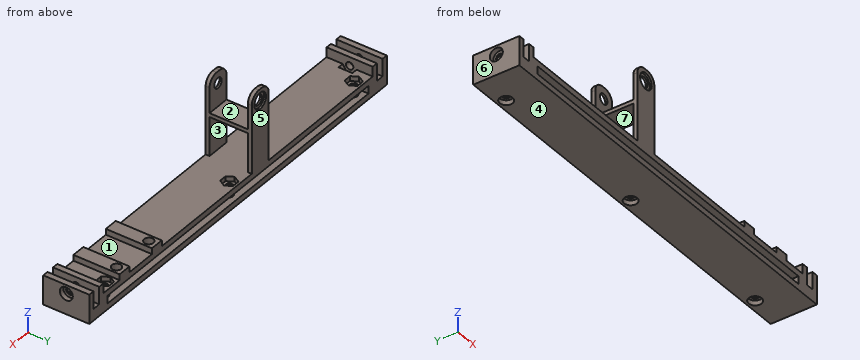
```python
from build123d import *

# Parameters (mm, degrees)
SKETCH2_W            = 23.75
SKETCH2_H            = 12
BOSS_EXTRUDE1_DEPTH  = 10
SKETCH3_W            = 12
SKETCH3_H            = 2.025
BOSS_EXTRUDE2_DEPTH  = 40
FILLET1_R            = 5
FILLET1_OF_MIRROR1_R = 5
SKETCH5_R            = 2.65
CUT_EXTRUDE1_DEPTH   = 57.639760769
SKETCH6_R            = 4.15
CUT_EXTRUDE2_DEPTH   = 1
SKETCH7_W            = 84
SKETCH7_H            = 23.75
SKETCH7_W_2          = 115.5
BOSS_EXTRUDE3_DEPTH  = 10
SKETCH8_W            = 10
SKETCH8_H            = 23.75
BOSS_EXTRUDE4_DEPTH  = 5
BOSS_EXTRUDE7_REACH  = 130.079
SKETCH18_W           = 12
SKETCH18_H           = 2
SKETCH11_W           = 185.5
SKETCH11_H           = 4
CUT_EXTRUDE3_DEPTH   = 9
SKETCH12_R           = 1.9
CUT_EXTRUDE4_DEPTH   = 155.807138078
SKETCH15_R           = 3.35
CUT_EXTRUDE5_DEPTH   = 2.5
SKETCH16_R           = 1.9
CUT_EXTRUDE6_DEPTH   = 2.5
LPATTERN1_COUNT      = 3
LPATTERN1_PITCH      = 88.5
SKETCH14_W           = 7
SKETCH14_H           = 23.75
BOSS_EXTRUDE6_DEPTH  = 3
CUT_EXTRUDE7_REACH   = 130.079
SKETCH21_W           = 4
SKETCH21_H           = 9
LPATTERN2_COUNT      = 2
LPATTERN2_PITCH      = 201.5
SKETCH22_R           = 2.4
CUT_EXTRUDE8_DEPTH   = 3.8
SKETCH26_R           = 1.75
CUT_EXTRUDE12_DEPTH  = 0.6
LPATTERN3_COUNT      = 2
LPATTERN3_PITCH      = 23
SKETCH23_R           = 1.9
CUT_EXTRUDE9_DEPTH   = 10
SKETCH24_R           = 3.35
CUT_EXTRUDE10_DEPTH  = 2.5
CUT_EXTRUDE11_DEPTH  = 3


with BuildPart() as part:
    # Sketch2 → Boss-Extrude1 (new body)
    with BuildSketch(Plane(origin=(0, 0, 0), x_dir=(0, 1, 0), z_dir=(0, 0, 1))):
        with Locations((-83.125, 6)):
            Rectangle(SKETCH2_W, SKETCH2_H)
    extrude(amount=BOSS_EXTRUDE1_DEPTH)

    # Sketch3 → Boss-Extrude2 (add)
    with BuildSketch(Plane.XY.offset(10)):
        with Locations((-6, -72.2625)):
            Rectangle(SKETCH3_W, SKETCH3_H)
    boss_extrude2 = extrude(amount=BOSS_EXTRUDE2_DEPTH)

    # Fillet1
    fillet1_edges = [part.edges().sort_by_distance(p)[0] for p in [
        (-12, -72.2625, 50),
        (0, -72.2625, 50),
    ]]
    fillet(fillet1_edges, radius=FILLET1_R)

    # Mirror1: Boss-Extrude2 across plane
    add(boss_extrude2.mirror(Plane.ZX.offset(-83.125)))

    # Fillet1 of Mirror1
    fillet1_of_mirror1_edges = [part.edges().sort_by_distance(p)[0] for p in [
        (-12, -93.9875, 50),
        (0, -93.9875, 50),
    ]]
    fillet(fillet1_of_mirror1_edges, radius=FILLET1_OF_MIRROR1_R)

    # Sketch5 → Cut-Extrude1 (cut, through all)
    with BuildSketch(Plane.XZ.offset(95)):
        with Locations(Location((-6, 44, 0), (0, 0, 270))):
            Circle(SKETCH5_R)
    extrude(amount=-CUT_EXTRUDE1_DEPTH, mode=Mode.SUBTRACT)

    # Sketch6 → Cut-Extrude2 (cut)
    with BuildSketch(Plane.XZ.offset(95)):
        with Locations(Location((-6, 44, 0), (0, 0, 270))):
            Circle(SKETCH6_R)
    cut_extrude2 = extrude(amount=-CUT_EXTRUDE2_DEPTH, mode=Mode.SUBTRACT)

    # Mirror2: Cut-Extrude2 across plane
    add(cut_extrude2.mirror(Plane.ZX.offset(-83.125)), mode=Mode.SUBTRACT)

    # Sketch7 → Boss-Extrude3 (add)
    with BuildSketch(Plane(origin=(0, 0, 0), x_dir=(1, 0, 0), z_dir=(0, 0, -1))):
        with Locations((-54, 83.125)):
            Rectangle(SKETCH7_W, SKETCH7_H)
        with Locations((57.75, 83.125)):
            Rectangle(SKETCH7_W_2, SKETCH7_H)
    extrude(amount=-BOSS_EXTRUDE3_DEPTH)

    # Sketch8 → Boss-Extrude4 (add)
    with BuildSketch(Plane.XY.offset(10)):
        with Locations((110.5, -83.125)):
            Rectangle(SKETCH8_W, SKETCH8_H)
        with Locations((-91, -83.125)):
            Rectangle(SKETCH8_W, SKETCH8_H)
    extrude(amount=BOSS_EXTRUDE4_DEPTH)

    # Sketch18 → Boss-Extrude7 (add, up to next)
    with BuildSketch(Plane(origin=(0, -71.25, 0), x_dir=(-1, 0, 0), z_dir=(0, 1, 0)), mode=Mode.PRIVATE) as boss_extrude7_sk1:
        with Locations((6, 31)):
            Rectangle(SKETCH18_W, SKETCH18_H)
    boss_extrude7_tool1 = extrude(boss_extrude7_sk1.sketch, amount=-BOSS_EXTRUDE7_REACH, mode=Mode.PRIVATE) - part.part
    add(boss_extrude7_tool1.solids().sort_by_distance((-6, -71.25, 31))[0])

    # Sketch11 → Cut-Extrude3 (cut)
    with BuildSketch(Plane(origin=(0, -71.25, 0), x_dir=(-1, 0, 0), z_dir=(0, 1, 0))):
        with Locations((-9.75, 5)):
            Rectangle(SKETCH11_W, SKETCH11_H)
    cut_extrude3 = extrude(amount=-CUT_EXTRUDE3_DEPTH, mode=Mode.SUBTRACT)

    # Mirror3: Cut-Extrude3 across plane
    add(cut_extrude3.mirror(Plane.ZX.offset(-83.125)), mode=Mode.SUBTRACT)

    # Sketch12 → Cut-Extrude4 (cut, symmetric)
    with BuildSketch(Plane.XY.offset(10)):
        with Locations((-78.75, -75.75)):
            Circle(SKETCH12_R)
    cut_extrude4 = extrude(amount=CUT_EXTRUDE4_DEPTH, both=True, mode=Mode.SUBTRACT)

    # Sketch15 → Cut-Extrude5 (cut)
    with BuildSketch(Plane.XY):
        with Locations((-78.75, -75.75)):
            Circle(SKETCH15_R)
    cut_extrude5 = extrude(amount=CUT_EXTRUDE5_DEPTH, mode=Mode.SUBTRACT)

    # Sketch16 → Cut-Extrude6 (cut)
    # profile 1 of 2: a face of its own
    with BuildSketch(Plane.XY.offset(10)):
        Polygon((-76.826794919, -72.418911087), (-80.673205081, -72.418911087), (-82.596410162, -75.75), (-80.673205081, -79.081088913), (-76.826794919, -79.081088913), (-74.903589838, -75.75), align=None)
        Polygon((-80.5, -72.718911087), (-82.25, -75.75), (-80.5, -78.781088913), (-77, -78.781088913), (-75.25, -75.75), (-77, -72.718911087), align=None, mode=Mode.SUBTRACT)
    # profile 2 of 2: a face of its own
    with BuildSketch(Plane.XY.offset(10)):
        Polygon((-77, -72.718911087), (-80.5, -72.718911087), (-82.25, -75.75), (-80.5, -78.781088913), (-77, -78.781088913), (-75.25, -75.75), align=None)
        with Locations((-78.75, -75.75)):
            Circle(SKETCH16_R, mode=Mode.SUBTRACT)
    cut_extrude6 = extrude(amount=-CUT_EXTRUDE6_DEPTH, mode=Mode.SUBTRACT)

    # LPattern1: Cut-Extrude4, Cut-Extrude5, Cut-Extrude6 ×3
    with Locations(*[(i * LPATTERN1_PITCH, 0, 0) for i in range(1, LPATTERN1_COUNT)]):
        add(cut_extrude4, mode=Mode.SUBTRACT)
        add(cut_extrude5, mode=Mode.SUBTRACT)
        add(cut_extrude6, mode=Mode.SUBTRACT)

    # Sketch14 → Boss-Extrude6 (add)
    with BuildSketch(Plane.XY.offset(10)):
        with Locations((67.5, -83.125)):
            Rectangle(SKETCH14_W, SKETCH14_H)
        with Locations((90.5, -83.125)):
            Rectangle(SKETCH14_W, SKETCH14_H)
    extrude(amount=BOSS_EXTRUDE6_DEPTH)

    # Sketch21 → Cut-Extrude7 (cut, up to next)
    with BuildSketch(Plane(origin=(0, -71.25, 0), x_dir=(-1, 0, 0), z_dir=(0, 1, 0)), mode=Mode.PRIVATE) as cut_extrude7_sk1:
        with Locations((-110.5, 10.5)):
            Rectangle(SKETCH21_W, SKETCH21_H)
    cut_extrude7_tool1 = extrude(cut_extrude7_sk1.sketch, amount=-CUT_EXTRUDE7_REACH, mode=Mode.PRIVATE) & part.part
    cut_extrude7 = cut_extrude7_tool1.solids().sort_by_distance((110.5, -71.25, 10.5))[0]
    add(cut_extrude7, mode=Mode.SUBTRACT)

    # LPattern2: Cut-Extrude7 ×2
    with Locations(*[(-i * LPATTERN2_PITCH, 0, 0) for i in range(1, LPATTERN2_COUNT)]):
        add(cut_extrude7, mode=Mode.SUBTRACT)

    # Sketch22 → Cut-Extrude8 (cut)
    with BuildSketch(Plane.XY.offset(13)):
        with Locations((90.5, -75.37)):
            Circle(SKETCH22_R)
    cut_extrude8 = extrude(amount=-CUT_EXTRUDE8_DEPTH, mode=Mode.SUBTRACT)

    # Sketch26 → Cut-Extrude12 (cut)
    with BuildSketch(Plane.XY.offset(9.2)):
        with Locations((90.5, -75.37)):
            Circle(SKETCH26_R)
    cut_extrude12 = extrude(amount=-CUT_EXTRUDE12_DEPTH, mode=Mode.SUBTRACT)

    # LPattern3: Cut-Extrude8, Cut-Extrude12 ×2
    with Locations(*[(-i * LPATTERN3_PITCH, 0, 0) for i in range(1, LPATTERN3_COUNT)]):
        add(cut_extrude8, mode=Mode.SUBTRACT)
        add(cut_extrude12, mode=Mode.SUBTRACT)

    # Sketch23 → Cut-Extrude9 (cut)
    with BuildSketch(Plane.YZ.offset(115.5)):
        with Locations(Location((-83.125, 10.5, 0), (0, 0, 270))):
            Circle(SKETCH23_R)
    cut_extrude9 = extrude(amount=-CUT_EXTRUDE9_DEPTH, mode=Mode.SUBTRACT)

    # Sketch24 → Cut-Extrude10 (cut)
    with BuildSketch(Plane.YZ.offset(115.5)):
        with Locations(Location((-83.125, 10.5, 0), (0, 0, 270))):
            Circle(SKETCH24_R)
    cut_extrude10 = extrude(amount=-CUT_EXTRUDE10_DEPTH, mode=Mode.SUBTRACT)

    # Sketch25 → Cut-Extrude11 (cut)
    with BuildSketch(Plane(origin=(105.5, 0, 0), x_dir=(0, -1, 0), z_dir=(-1, 0, 0))):
        Polygon((81.201794919, 13.831088913), (79.278589838, 10.5), (81.201794919, 7.168911087), (85.048205081, 7.168911087), (86.971410162, 10.5), (85.048205081, 13.831088913), align=None)
    cut_extrude11 = extrude(amount=CUT_EXTRUDE11_DEPTH, mode=Mode.SUBTRACT)

    # Mirror4: Cut-Extrude9, Cut-Extrude10, Cut-Extrude11 across plane
    add(cut_extrude9.mirror(Plane(origin=(9.75, 0, 0), x_dir=(0, 0, 1), z_dir=(1, 0, 0))), mode=Mode.SUBTRACT)
    add(cut_extrude10.mirror(Plane(origin=(9.75, 0, 0), x_dir=(0, 0, 1), z_dir=(1, 0, 0))), mode=Mode.SUBTRACT)
    add(cut_extrude11.mirror(Plane(origin=(9.75, 0, 0), x_dir=(0, 0, 1), z_dir=(1, 0, 0))), mode=Mode.SUBTRACT)


solid = part.part
```
Read the model definition and answer for the solid it produces. Units are mm, in the model's axes. Face numbers are marked on the shaded views. A direction names the side the tool comes from. Coordinates: 2 decimals unless noted, no trailing zeros. Write each loop counter-clockwise with the first axis right and the second up, starting at its lowest first coordinate (ties: lowest second). Pieces come first, ordered by that corner, then holes. Notation, with made-up numbers: (41.5, 9) -> (57.5, 9) arc R5 cw to (57.5, 13) -> close; hole circle Ø11 at (-26.5, 23). An arc over 180 degrees is marked (long way). Return JSON: item names as keys, results as strings.
1. A cutting plane is placed at C-C (x = -59). Determine the outline of the cut face in (y, z).
Found:
{"outline": "(-95, 0) -> (-71.25, 0) -> (-71.25, 3) -> (-80.25, 3) -> (-80.25, 7) -> (-71.25, 7) -> (-71.25, 10) -> (-95, 10) -> (-95, 7) -> (-86, 7) -> (-86, 3) -> (-95, 3) -> close"}
2. A cutting plane is placed at A-A (y = -90). Give the number of separate pieces and of enclosed holes in the cut face, and give its area (3 significant figures).
Found:
{"separate pieces": "2", "enclosed holes": "1", "area": "1,470 mm2"}
3. A cutting plane is placed at D-D (x = 90.5). Determine the outline of the cut face in (y, z), and give its area (3 significant figures).
Found:
{"outline": "(-95, 0) -> (-71.25, 0) -> (-71.25, 3) -> (-80.25, 3) -> (-80.25, 7) -> (-71.25, 7) -> (-71.25, 13) -> (-72.97, 13) -> (-72.97, 9.2) -> (-73.62, 9.2) -> (-73.62, 8.6) -> (-77.12, 8.6) -> (-77.12, 9.2) -> (-77.77, 9.2) -> (-77.77, 13) -> (-95, 13) -> (-95, 7) -> (-86, 7) -> (-86, 3) -> (-95, 3) -> close", "area": "216 mm2"}
4. Find the intervals of material crossed by line 1 along X through (y, z) = (-75.75, 7.1); line 2 along Z through (x, y) = (1, -92); line 3 along Y through (x, z) = (107.55, 10.5) (3 decimals), in increasing order. Write a range as from..to.
Found:
{"line 1": "-96..-93, -89..-80.65, -76.85..7.85, 11.65..96.35, 100.15..108.5, 112.5..115.5", "line 2": "0..3, 7..10", "line 3": "-95..-85.025, -81.225..-71.25"}
5. Determine the mould class of the marked faces 5, 6 and 7 for opening direction Y: pulls with the +Y half, pulls with the -Y half, needs draft (parallel to the pull), parting line crosses it, or undercut.
Found:
{"face 5": "pulls with the +Y half", "face 6": "needs draft", "face 7": "undercut"}
6. A tool of negligible diameter and unlimited length cuts with its end or side. For the marked faces 1, 2, 3 and 4, from which of +Z, -Z, +X, -X, +Y, -Y can it reach the whole face along a straight path? Write none if from no direction.
Found:
{"face 1": "+Z, +Y, -Y", "face 2": "+Z, +X, -X", "face 3": "none", "face 4": "-Z, +X, -X, +Y, -Y"}
7. A cutting plane is placed at B-B (z = 24.5). Determine the outline of the cut face in (x, y) (3 decimals).
Found:
{"outline": "(-12, -95) -> (0, -95) -> (0, -92.975) -> (-12, -92.975) -> close; (-12, -73.275) -> (0, -73.275) -> (0, -71.25) -> (-12, -71.25) -> close"}
8. Each of these flat-tipped pins is pushed along its axis until it touches: P1, Ø10, axis at y = -92, z = 36.5, coming from the -X side; P2, Ø4, axis at x = -78.75, y = -75.75, coming from the +Z side; P3, Ø2.5, axis at y = -83.125, z = 10.5, coming from the -X side; P4, Ø7, axis at y = -83.5, z = 12.5, coming from the -X side. Where does it stop, or does it pass through?
Found:
{"P1": "x = -12", "P2": "z = 7.5", "P3": "x = -83", "P4": "x = -96"}
